from build123d import *

# Parameters (mm, degrees)
F0_W      = 203.2
F0_H      = 38.1
F1_DEPTH  = 25.4
F2_W      = 196.85
F2_H      = 44.45
F3_DEPTH  = 34.925
F4_R      = 1.5875
F5_DEPTH  = 50.8
F6_W      = 185.9018951654
F6_H      = 9.962297976
F7_DEPTH  = 19.05
F8_R      = 5.08
F9_SIZE   = 0.635
F10_R     = 1.27
F11_R     = 2.54
F12_DEPTH = 5.08


with BuildPart() as f1:
    # F0 (on Front) → F1 (new body, symmetric)
    with BuildSketch(Plane.XZ):
        Rectangle(F0_W, F0_H)
    extrude(amount=F1_DEPTH, both=True)

    # F2 (on face) → F3 (cut)
    with BuildSketch(Plane.XY.offset(19.05)):
        Rectangle(F2_W, F2_H)
    extrude(amount=-F3_DEPTH, mode=Mode.SUBTRACT)

    # F4 (on face) → F5 (join)
    with BuildSketch(Plane.XY.offset(-15.875)):
        Circle(F4_R)
        with Locations((-38.1, 0)):
            Circle(F4_R)
        with Locations((-76.2, 0)):
            Circle(F4_R)
        with Locations((38.1, 0)):
            Circle(F4_R)
        with Locations((76.2, 0)):
            Circle(F4_R)
    extrude(amount=F5_DEPTH)

    # F6 (on face) → F7 (cut)
    with BuildSketch(Plane.XY.offset(19.05)):
        with Locations((0, -23.8689258695)):
            Rectangle(F6_W, F6_H)
    extrude(amount=-F7_DEPTH, mode=Mode.SUBTRACT)

    # F8
    f8_edges = [f1.edges().sort_by_distance(p)[0] for p in [
        (-92.950948, -23.8125, 19.05),
        (-92.950948, -23.8125, 0),
        (92.950948, -23.8125, 19.05),
        (92.950948, -23.8125, 0),
    ]]
    fillet(f8_edges, radius=F8_R)

    # F9
    f9_edges = [f1.edges().sort_by_distance(p)[0] for p in [
        (-1.5875, 0, 34.925),
        (-39.6875, 0, 34.925),
        (36.5125, 0, 34.925),
        (74.6125, 0, 34.925),
        (-77.7875, 0, 34.925),
    ]]
    chamfer(f9_edges, length=F9_SIZE)

    # F10
    f10_edges = [f1.edges().sort_by_distance(p)[0] for p in [
        (0, 22.225, 19.05),
        (-98.425, 0, 19.05),
        (0, -25.4, 0),
        (-91.46305, -25.4, 1.487898),
        (-92.950948, -25.4, 9.525),
        (-99.815474, -25.4, 19.05),
        (-101.6, 0, 19.05),
        (101.6, 0, 19.05),
        (101.6, -25.4, 0),
        (0, -25.4, -19.05),
        (101.6, 0, -19.05),
        (-101.6, -25.4, 0),
        (-101.6, 0, -19.05),
        (0, 22.225, -15.875),
        (0, -22.225, 0),
        (98.425, 0, 19.05),
        (98.425, 0, -15.875),
    ]]
    fillet(f10_edges, radius=F10_R)

    # F11 (on face) → F12 (cut)
    with BuildSketch(Plane.XZ.offset(-22.225)):
        with Locations((55.88, 7.5767044909)):
            Circle(F11_R)
        with Locations((-55.88, 7.5767044909)):
            Circle(F11_R)
    extrude(amount=-F12_DEPTH, mode=Mode.SUBTRACT)


solid = f1.part
The listing builds one solid part. Answer for the finished solid, in the listing's coordinates (mm). A direction names the side the tool comes from. Coordinates: 2 decimals unless noted, no trailing zeros. Write each loop counter-clockwise with the first axis right and the second up, starting at its lowest first coordinate (ties: lowest second). Pieces come first, ordered by that corner, then holes. Notation, with made-up numbers: (33, 52.5) - (76, 52.5) arc R20 cw to (76, 77.5) - close; hole circle Ø9 at (-9, 64). An arc over 180 degrees is marked (long way). Put each result on its own line as item: value.
1. The part is cut by section D-D on x = 64. Give the vertices of the cut face in (y, z) (3 decimals).
Answer sheet:
outline: (-25.4, -17.78) arc R1.27 ccw to (-24.13, -19.05) - (25.4, -19.05) - (25.4, 19.05) - (23.495, 19.05) arc R1.27 ccw to (22.225, 17.78) - (22.225, -14.605) arc R1.27 cw to (20.955, -15.875) - (-22.225, -15.875) - (-22.225, -1.27) arc R1.27 ccw to (-23.495, 0) - (-24.13, 0) arc R1.27 ccw to (-25.4, -1.27) - close
2. The part is cut by section C-C on y = -14. Give the vertices of the cut face in (x, z) (3 decimals).
Answer sheet:
outline: (-101.6, -17.78) arc R1.27 ccw to (-100.33, -19.05) - (100.33, -19.05) arc R1.27 ccw to (101.6, -17.78) - (101.6, 17.78) arc R1.27 ccw to (100.33, 19.05) - (99.695, 19.05) arc R1.27 ccw to (98.425, 17.78) - (98.425, -14.605) arc R1.27 cw to (97.155, -15.875) - (-98.425, -15.875) - (-98.425, 17.78) arc R1.27 ccw to (-99.695, 19.05) - (-100.33, 19.05) arc R1.27 ccw to (-101.6, 17.78) - close
3. The part is cut by section B-B on z = 23.5. Give the vertices of the cut face in (x, y) (1 decimal), plus the area to 3 significant figures.
Answer sheet:
outline: circle Ø3.2 at (-76.2, 0); circle Ø3.2 at (-38.1, 0); circle Ø3.2 at (0, 0); circle Ø3.2 at (38.1, 0); circle Ø3.2 at (76.2, 0)
area: 39.6 mm^2
4. Find the intervals of material crossed by line 1 along X through (y, z) = (-10, 14.5) (3 decimals); line 2 along Z through (x, y) = (-55.88, 24.7); line 3 along Y through (x, z) = (-58, -6.5) (3 decimals), in increasing order. Write a range as from..to.
Answer sheet:
line 1: x = -101.6..-98.425, 98.425..101.6
line 2: z = -19.05..5.04, 10.12..19.05
line 3: y = -25.4..-22.225, 22.225..25.4
5. Determine the mould class of faces 1 (the face through (101.6, 0, 0)), 2 (the face through (-91.502, -23.808, 1.528)), 3 (the face through (53.342, 23.79, 7.688)) for opening direction Z: pulls with the +Z half, pulls with the -Z half, needs draft (parallel to the pull), parting line crosses it, or undercut.
Answer sheet:
face 1: needs draft
face 2: pulls with the +Z half
face 3: undercut
6. Flat-ended cylindrical pins translate along their axes: pin 1 Ø1.5 at (x, z) = (-73, 18.5) entering from -Y (3 decimals); pin 2 Ø10 at (x, y) = (-5, -15) entering from +Z (3 decimals); pin 3 Ø5 at (x, z) = (38, 29.5) entering from +Y. Find the tip coordinate at first contact, or state that the pin passes through.
Answer sheet:
pin 1: stops at y = 22.225
pin 2: stops at z = -15.875
pin 3: stops at y = 1.59
7. A tool of negligible diameter and unlimited length cuts with its end or side. For faces 4 (the face through (-1, 0, -19.05)), 5 (the face through (-94.48, -23.81, 17.6)), 6 (the face through (-1, 22.225, 2)), from which of +Z, -Z, +X, -X, +Y, -Y can it reach the whole face along a straight path? Write none if from no direction.
Answer sheet:
face 4: -Z, +X, -X, +Y, -Y
face 5: +Z, -Y
face 6: +Z
8. The part is cut by section A-A on x = -55.88. Give the vertices of the cut face in (y, z) (3 decimals), plus the area to 3 significant figures.
Answer sheet:
outline: (-25.4, -17.78) arc R1.27 ccw to (-24.13, -19.05) - (25.4, -19.05) - (25.4, 5.037) - (22.225, 5.037) - (22.225, -14.605) arc R1.27 cw to (20.955, -15.875) - (-22.225, -15.875) - (-22.225, -1.27) arc R1.27 ccw to (-23.495, 0) - (-24.13, 0) arc R1.27 ccw to (-25.4, -1.27) - close; (22.225, 10.117) - (25.4, 10.117) - (25.4, 19.05) - (23.495, 19.05) arc R1.27 ccw to (22.225, 17.78) - close
area: 305 mm^2
